Could you check a few things on this model? Use its own coordinates, in mm. Round coordinates to 2 decimals unless told otherwise and drop trailing zeros. Loops run counter-clockwise (first coordinate to the right, second up) from the corner with the lowest first, then second, coordinate; pieces in that order, holes last. Notation, with made-up numbers: (-34.75, 34.5) -> (-27.75, 34.5) arc R12 cw to (-27.75, 46.5) -> close; hole circle Ø7 at (45.25, 6.25). An arc over 180 degrees is marked (long way). Write each question's results on one line, items separated by ' | '. Start each with the question number.
1) For P1, Ø10, axis at x = 791, y = 1049, coming from the -Z side; P2, Ø2.5, axis at x = 784.69, y = 1089.39, coming from the -Z side, each with a flat end and sliding along its axis, tell me the tip position at first contact or that it passes through.
2) Imagine slicing it at B-B, the plane x = 897. List the corners of the cut face in (y, z) for me.
3) If I drill on probe 1 along Y at (x, z) = (783.5, 0.75); probe 2 along X at (y, z) = (1090, 0.5); probe 3 along Y at (x, z) = (778.5, 3.25), over which ranges is the centre line in solid material (lowest first)?
4) Imagine slicing it at A-A, the plane z = 4.05. List the corners of the cut face in (x, y) for me.
from build123d import *

# Parameters (mm, degrees)
SKETCH2_R           = 1.5
BOSS_EXTRUDE1_DEPTH = 5


with BuildPart() as part:
    # Sketch2 → Boss-Extrude1 (new body)
    with BuildSketch(Plane.XY):
        with BuildLine():
            Line((792.944636851, 1099.1431403), (882.944636851, 1099.1431403))
            Line((882.944636851, 1099.1431403), (891.194636851, 1099.1431403))
            ThreePointArc((891.194636851, 1099.1431403), (901.801238569, 1094.749742018), (906.194636851, 1084.1431403))
            Line((906.194636851, 1084.1431403), (906.194636851, 1018.1431403))
            ThreePointArc((906.194636851, 1018.1431403), (901.801238569, 1007.536538582), (891.194636851, 1003.1431403))
            Line((891.194636851, 1003.1431403), (784.694636851, 1003.1431403))
            ThreePointArc((784.694636851, 1003.1431403), (774.088035133, 1007.536538582), (769.694636851, 1018.1431403))
            Line((769.694636851, 1018.1431403), (769.694636851, 1084.1431403))
            ThreePointArc((769.694636851, 1084.1431403), (774.088035133, 1094.749742018), (784.694636851, 1099.1431403))
            Line((784.694636851, 1099.1431403), (792.944636851, 1099.1431403))
        make_face()
        with Locations((784.694636851, 1089.3931403)):
            Circle(SKETCH2_R, mode=Mode.SUBTRACT)
        with Locations((784.694636851, 1012.8931403)):
            Circle(SKETCH2_R, mode=Mode.SUBTRACT)
        with Locations((891.194636851, 1012.8931403)):
            Circle(SKETCH2_R, mode=Mode.SUBTRACT)
        with Locations((891.194636851, 1089.3931403)):
            Circle(SKETCH2_R, mode=Mode.SUBTRACT)
    extrude(amount=BOSS_EXTRUDE1_DEPTH)


solid = part.part
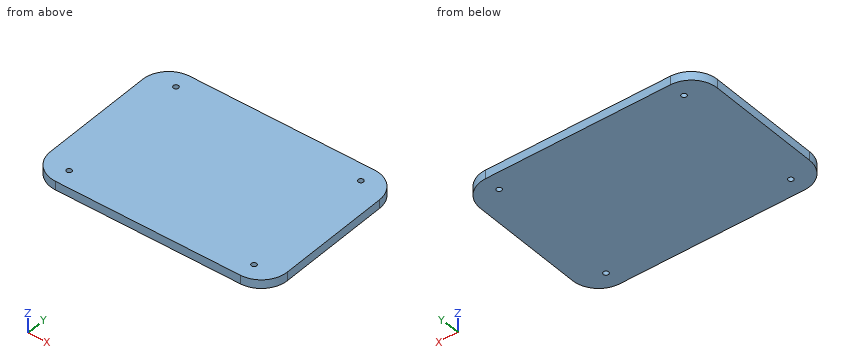
Checked values:
1) P1: z = 0 | P2: through
2) outline: (1004.31, 0) -> (1097.97, 0) -> (1097.97, 5) -> (1004.31, 5) -> close
3) probe 1: 1003.19 to 1011.99, 1013.8 to 1088.49, 1090.3 to 1099.1 | probe 2: 770.89 to 783.32, 786.07 to 889.82, 892.57 to 905 | probe 3: 1004.48 to 1097.8
4) outline: (769.69, 1018.14) arc R15 ccw to (784.69, 1003.14) -> (891.19, 1003.14) arc R15 ccw to (906.19, 1018.14) -> (906.19, 1084.14) arc R15 ccw to (891.19, 1099.14) -> (784.69, 1099.14) arc R15 ccw to (769.69, 1084.14) -> close; hole circle Ø3 at (784.69, 1012.89); hole circle Ø3 at (784.69, 1089.39); hole circle Ø3 at (891.19, 1012.89); hole circle Ø3 at (891.19, 1089.39)
